from build123d import *

# Parameters (mm, degrees)
SKETCH_1_W                = 2000
SKETCH_1_H                = 270
EXTRUDE_1_DEPTH           = 5
HOLE_WIZARD_1_D           = 6.6
HOLE_WIZARD_1_CBORE_D     = 11
HOLE_WIZARD_1_CBORE_DEPTH = 6.8
HOLE_WIZARD_M10_1_D       = 8.5
HOLE_WIZARD_9_0_9_3_D     = 9
HOLE_WIZARD_9_0_9_4_D     = 9
HOLE_WIZARD_11_0_11_1_D   = 11
SKETCH_20_R               = 30
CUT_EXTRUDE_1_DEPTH       = 11
HOLE_WIZARD_5_D           = 6.6
HOLE_WIZARD_5_CBORE_D     = 11
HOLE_WIZARD_5_CBORE_DEPTH = 6.8
HOLE_WIZARD_6_D           = 6.6
HOLE_WIZARD_6_CBORE_D     = 11
HOLE_WIZARD_6_CBORE_DEPTH = 6.8


with BuildPart() as part:
    # 草图1 → 凸台-拉伸1 (new body, symmetric)
    with BuildSketch(Plane.XY):
        Rectangle(SKETCH_1_W, SKETCH_1_H)
    extrude(amount=EXTRUDE_1_DEPTH, both=True)

    # 打孔尺寸(%根据)内六角圆柱头螺钉的类型1 (through all)
    with Locations(Plane(origin=(-992.5, 125, 5), x_dir=(1, 0, 0), z_dir=(0, 0, 1))):
        with Locations((0, 0), (0, -250), (1985, 0), (1985, -250), (1985, -125), (0, -125)):
            CounterBoreHole(HOLE_WIZARD_1_D / 2, HOLE_WIZARD_1_CBORE_D / 2, HOLE_WIZARD_1_CBORE_DEPTH)

    # M10 螺纹孔1 (through all)
    with Locations(Plane(origin=(952.5, -120, 5), x_dir=(1, 0, 0), z_dir=(0, 0, 1))):
        with Locations((0, 0), (0, 30)):
            hole_wizard_m10_1 = Hole(HOLE_WIZARD_M10_1_D / 2)

    # Ø9.0 (9) 直径孔3 (through all)
    with Locations(Plane(origin=(-345, -68, -5), x_dir=(-1, 0, 0), z_dir=(0, 0, -1))):
        with Locations((0, 0), (0, -30), (510, 0), (510, -30)):
            Hole(HOLE_WIZARD_9_0_9_3_D / 2)

    # Ø9.0 (9) 直径孔4 (through all)
    with Locations(Plane(origin=(-555, 7, -5), x_dir=(-1, 0, 0), z_dir=(0, 0, -1))):
        with Locations((0, 0), (90, 0), (90, -60), (0, -60)):
            Hole(HOLE_WIZARD_9_0_9_4_D / 2)

    # Ø11.0 (11) 直径孔1 (through all)
    with Locations(Plane(origin=(36, -8, -5), x_dir=(-1, 0, 0), z_dir=(0, 0, -1))):
        with Locations((0, 0), (72, 0), (72, 72), (0, 72)):
            Hole(HOLE_WIZARD_11_0_11_1_D / 2)

    # 草图20 → 切除-拉伸1 (cut, through all)
    with BuildSketch(Plane(origin=(0, 0, -5), x_dir=(-1, 0, 0), z_dir=(0, 0, -1))):
        with Locations((0, 28)):
            Circle(SKETCH_20_R)
    extrude(amount=-CUT_EXTRUDE_1_DEPTH, mode=Mode.SUBTRACT)

    # 打孔尺寸(%根据)内六角圆柱头螺钉的类型5 (through all)
    with Locations(Plane(origin=(-900, 95, 5), x_dir=(1, 0, 0), z_dir=(0, 0, 1))):
        with Locations((0, 0), (300, 0), (600, 0), (900, 0), (1200, 0), (1500, 0), (1800, 0)):
            CounterBoreHole(HOLE_WIZARD_5_D / 2, HOLE_WIZARD_5_CBORE_D / 2, HOLE_WIZARD_5_CBORE_DEPTH)

    # 镜向1: M10 螺纹孔1 across plane
    add(hole_wizard_m10_1.mirror(Plane(origin=(0, 0, 0), x_dir=(0, 0, 1), z_dir=(1, 0, 0))), mode=Mode.SUBTRACT)

    # 打孔尺寸(%根据)内六角圆柱头螺钉的类型6 (through all)
    with Locations(Plane(origin=(907.5, -70, 5), x_dir=(1, 0, 0), z_dir=(0, 0, 1))):
        with Locations((0, 0), (60, 0)):
            hole_wizard_6 = CounterBoreHole(HOLE_WIZARD_6_D / 2, HOLE_WIZARD_6_CBORE_D / 2, HOLE_WIZARD_6_CBORE_DEPTH)

    # 镜向2: 打孔尺寸(%根据)内六角圆柱头螺钉的类型6 across plane
    add(hole_wizard_6.mirror(Plane(origin=(0, 0, 0), x_dir=(0, 0, 1), z_dir=(1, 0, 0))), mode=Mode.SUBTRACT)


solid = part.part
Design review of the part built by this model. Coordinates are the model's own, in mm. Round coordinates to 2 decimals unless told otherwise and drop trailing zeros. Use a Markdown table: item, result. Add a question column.
1. Mouldability with a two-part tool opening along X and no side actions: class faces 1 (the face through (-14, -28, -5)), 2 (the face through (6.503, -1.287, -0.07)) as +X half, -X half, draft (parallel to the pull), parting line (faces both ways), or undercut.
2. Clearance check with flat-ended pins moving along their axes: pin 1 (9 mm diameter, centred on x = -967.5, y = -70, fed in from +Z); pin 2 (4 mm diameter, centred on x = 992.5, y = -125, fed in from -Z). State where each tip first meets the part, or that it passes through.
3. Wall thickness on probe 1 along Y at (x, z) = (-907.5, 3.25); probe 2 along Y at (x, z) = (-345, 0.25); probe 3 along X at (y, z) = (24.5, 3.75): over which ranges is each line inside the solid? List them lowest first.
Output:
| question | item | result |
|---|---|---|
| 1 | face 1 | draft |
| 1 | face 2 | undercut |
| 2 | pin 1 | stops at z = -1.8 |
| 2 | pin 2 | passes through |
| 3 | probe 1 | y = -135 to -75.5, -64.5 to 135 |
| 3 | probe 2 | y = -135 to -102.5, -93.5 to -72.5, -63.5 to 135 |
| 3 | probe 3 | x = -1000 to -29.8, 29.8 to 1000 |
